The model under review builds one solid part; all positions refer to its coordinate system, in mm. Face numbers are marked on the shaded views. Coordinates: 2 decimals unless noted, no trailing zeros. Write each loop counter-clockwise with the first axis right and the second up, starting at its lowest first coordinate (ties: lowest second). Pieces come first, ordered by that corner, then holes.
1) Add section A-A, the plane x = 13. State the section outline as (y, z) points, then the cut area to 3 significant figures.
2) Add section C-C, the plane y = 19.5. State the section outline as (x, z) points, then the cut area to 3 significant figures.
3) For P1, Ø10, axis at x = 40, z = 434, coming from the +Y side, flat-tipped, find the tip position at first contact; note if it passes through.
4) Add section D-D, the plane z = 85.5. State the section outline as (x, y) points.
5) Add section B-B, the plane z = 385. State the section outline as (x, y) points, then the cut area to 3 significant figures.
6) For line 1 (X direction, y = -2.55, z = 385); line 2 (Z direction, x = 12, y = 10); line 3 (Z direction, x = 25, y = -3.3), list the stretches that pass through material, from the lowest coordinate up.
7) Mouldability with a two-part tool opening along Z and no side actions: class the marked faces 1 and 2 as released by +Z, released by -Z, zero draft, split by the parting line, or undercut.
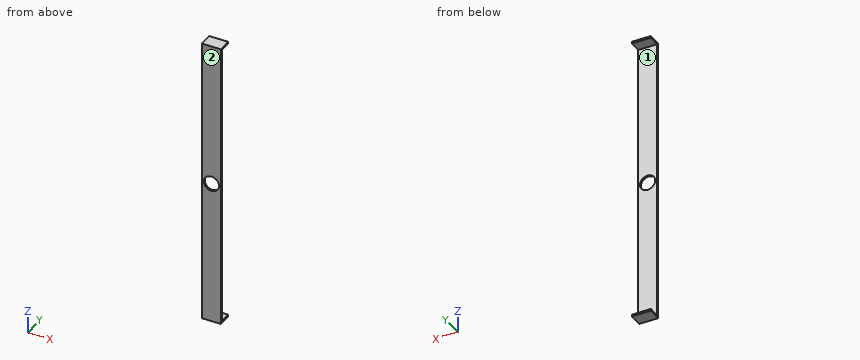
from build123d import *

# Parameters (mm, degrees)
SKETCH2_W           = 50
SKETCH2_H           = 5
BOSS_EXTRUDE1_DEPTH = 770
SKETCH3_W           = 50
SKETCH3_H           = 5
BOSS_EXTRUDE2_DEPTH = 30
SKETCH4_R           = 20
CUT_EXTRUDE1_DEPTH  = 30


with BuildPart() as part:
    # Sketch2 → Boss-Extrude1 (new body)
    with BuildSketch(Plane.XY):
        with Locations((25, -2.5)):
            Rectangle(SKETCH2_W, SKETCH2_H)
    extrude(amount=BOSS_EXTRUDE1_DEPTH)

    # Sketch3 → Boss-Extrude2 (add)
    with BuildSketch(Plane(origin=(0, 0, 0), x_dir=(1, 0, 0), z_dir=(0, 1, 0))):
        with Locations((25, -767.5)):
            Rectangle(SKETCH3_W, SKETCH3_H)
        with Locations((25, -2.5)):
            Rectangle(SKETCH3_W, SKETCH3_H)
    extrude(amount=BOSS_EXTRUDE2_DEPTH)

    # Sketch4 → Cut-Extrude1 (cut)
    with BuildSketch(Plane(origin=(0, 0, 0), x_dir=(1, 0, 0), z_dir=(0, 1, 0))):
        with Locations((25, -385)):
            Circle(SKETCH4_R)
    extrude(amount=-CUT_EXTRUDE1_DEPTH, mode=Mode.SUBTRACT)


solid = part.part
Geometry results:
1. outline: (-5, 0) - (30, 0) - (30, 5) - (0, 5) - (0, 369) - (-5, 369) - close; (-5, 401) - (0, 401) - (0, 765) - (30, 765) - (30, 770) - (-5, 770) - close
1. area: 3,990 mm2
2. outline: (0, 0) - (50, 0) - (50, 5) - (0, 5) - close; (0, 765) - (50, 765) - (50, 770) - (0, 770) - close
2. area: 500 mm2
3. P1: stops at y = 0
4. outline: (0, -5) - (50, -5) - (50, 0) - (0, 0) - close
5. outline: (0, -5) - (5, -5) - (5, 0) - (0, 0) - close; (45, -5) - (50, -5) - (50, 0) - (45, 0) - close
5. area: 50.0 mm2
6. line 1: x = 0 to 5, 45 to 50
6. line 2: z = 0 to 5, 765 to 770
6. line 3: z = 0 to 365, 405 to 770
7. face 1: undercut
7. face 2: zero draft
